```python
from build123d import *

# Parameters (mm, degrees)
F0_R     = 13.5
F1_DEPTH = 8
F2_R     = 12
F3_DEPTH = 7
F4_W     = 12
F4_H     = 11
F5_DEPTH = 0.7
F6_R     = 4
F7_DEPTH = 0.3


with BuildPart() as f1:
    # F0 (on Top) → F1 (new body)
    with BuildSketch(Plane.XY):
        Circle(F0_R)
    extrude(amount=F1_DEPTH)

    # F2 (on face) → F3 (cut)
    with BuildSketch(Plane(origin=(0, 0, 0), x_dir=(1, 0, 0), z_dir=(0, 0, -1))):
        Circle(F2_R)
    extrude(amount=-F3_DEPTH, mode=Mode.SUBTRACT)

    # F4 (on face) → F5 (cut)
    with BuildSketch(Plane.XY.offset(8)):
        with Locations((0.328328, 0.338116)):
            Rectangle(F4_W, F4_H)
    extrude(amount=-F5_DEPTH, mode=Mode.SUBTRACT)

    # F6 (on face) → F7 (cut)
    with BuildSketch(Plane.XY.offset(7.3)):
        Circle(F6_R)
    extrude(amount=-F7_DEPTH, mode=Mode.SUBTRACT)


solid = f1.part
```
Geometry: final body of the model. Coordinates: model frame, mm. A direction names the side the tool comes from. Coordinates: 2 decimals unless noted, no trailing zeros. Order: outer loops, then holes, each group sorted by start corner. A loop starts at its lowest first (then second) coordinate and runs counter-clockwise, first axis right, second up.
Item 1: Section query D-D (z = 1). Output: boundary loops of the cut face in (x, y).
Answer:
outline: circle Ø27 at (0, 0); hole circle Ø24 at (0, 0)
Item 2: Section query A-A (x = 0). Output: boundary loops of the cut face in (y, z), then the cut area to 3 significant figures.
Answer:
outline: (-13.5, 0) - (-12, 0) - (-12, 7) - (-4, 7) - (-4, 7.3) - (-5.16, 7.3) - (-5.16, 8) - (-13.5, 8) - close; (4, 7) - (12, 7) - (12, 0) - (13.5, 0) - (13.5, 8) - (5.84, 8) - (5.84, 7.3) - (4, 7.3) - close
area: 37.9 mm2
Item 3: Access query for faces 4 (the face through (3, 3, 7.3)), 5 (the face through (-11.99, -0.53, 3.45)), 6 (the face through (0, -6, 8)). Directions: +Z, -Z, +X, -X, +Y, -Y. A direction counts if a zero-diameter tool reaches every point of the face in a straight line with its end or side. Return the directions, or none.
Answer:
face 4: +Z
face 5: -Z
face 6: +Z, +X, -X, +Y, -Y
Item 4: Section query B-B (y = 0). Output: boundary loops of the cut face in (x, z), then the cut area to 3 significant figures.
Answer:
outline: (-13.5, 0) - (-12, 0) - (-12, 7) - (-4, 7) - (-4, 7.3) - (-5.67, 7.3) - (-5.67, 8) - (-13.5, 8) - close; (4, 7) - (12, 7) - (12, 0) - (13.5, 0) - (13.5, 8) - (6.33, 8) - (6.33, 7.3) - (4, 7.3) - close
area: 37.2 mm2
Item 5: Section query C-C (x = -11.5). Output: boundary loops of the cut face in (y, z).
Answer:
outline: (-7.07, 0) - (-3.43, 0) - (-3.43, 7) - (3.43, 7) - (3.43, 0) - (7.07, 0) - (7.07, 8) - (-7.07, 8) - close
Item 6: Contact query for flat-ended pins moving along their axis: P1, Ø9, axis at x = 0, y = 0, coming from the +Z side; P2, Ø2, axis at x = -7.5, z = 6.5, coming from the +Y side; P3, Ø0.6, axis at x = 1.5, z = 7.5, coming from the +Y side. Output: stop coordinate, or through.
Answer:
P1: stops at z = 7.3
P2: stops at y = 11.83
P3: stops at y = 13.45
Item 7: Material intervals for line 1 along Y through (x, z) = (0, 7.2); line 2 along Y through (x, z) = (0, 2); line 3 along Z through (x, y) = (9.75, 5.5), sorted ascending.
Answer:
line 1: y = -13.5 to -4, 4 to 13.5
line 2: y = -13.5 to -12, 12 to 13.5
line 3: z = 7 to 8
Item 8: Draft query along Y for faces 1 (the face through (-3, -3, 7)), 2 (the face through (-12, -2, 0)), 3 (the face through (-2.93, -13.18, 3.94)). Return one class per face: released by +Y, released by -Y, zero draft, split by the parting line, or undercut.
Answer:
face 1: undercut
face 2: zero draft
face 3: split by the parting line
